Can you work these out from the model? Positions are in its coordinate system, mm. Face numbers are marked on the shaded views. A direction names the side the tool comes from. Give positions to 0.01 mm unless a question says otherwise; leave off trailing zeros. Loops run counter-clockwise (first coordinate to the right, second up) from the corner with the lowest first, then second, coordinate; pieces in that order, holes last. Notation, with made-up numbers: (9, -28) - (52, -28) arc R22 cw to (52, -1) - close; hole circle Ø4 at (72, 23.25). An arc over 180 degrees is marked (long way). Answer as a JSON object with one key per item and string values. Group by question number.
Item 1: Suppose I cut it at D-D on y = 0. Write out the boundary of the cut face in (x, z), and give its area (3 significant figures).
Item 2: Suppose I cut it at C-C on x = 15. Write out the boundary of the cut face in (y, z), and give its area (3 significant figures).
Item 3: Please list where these lines run through material, in increasing order: L1, parallel to X at y = 0, z = 2.35; L2, parallel to Y at x = 5, z = 2.25; L3, parallel to Z at x = 18, y = -3.25.
Item 4: Which directions (+Z, -Z, +X, -X, +Y, -Y) give clear straight access to the entire face, cutting with the end or side of a thin tool? Please do the marked faces 5 and 6.
Item 5: Suppose I cut it at A-A on y = 8.75. Write out the boundary of the cut face in (x, z), and give its area (3 significant figures).
Item 6: Thinking about a two-plate mould opening in X: for the marked faces 1, 2, 3 and 4, which applies, pulls with the +X half, pulls with the -X half, needs draft (parallel to the pull), parting line crosses it, or undercut?
Item 7: Will these pins go through, and if not, where does the flat tip stop? pin 1 (7 mm diameter, centred on x = -4.5, y = -5.5, fed in from +Z); pin 2 (2 mm diameter, centred on x = -19.5, y = -12, fed in from +Z).
Item 8: Suppose I cut it at B-B on z = 3.2. Write out the boundary of the cut face in (x, y).
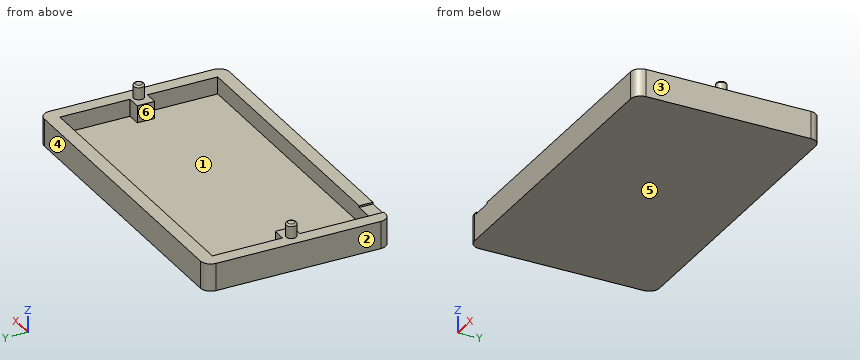
from build123d import *

# Parameters (mm, degrees)
SKETCH_W     = 46
SKETCH_H     = 27
PAD_DEPTH    = 2.5
SKETCH001_W  = 46
SKETCH001_H  = 27
PAD001_DEPTH = 1.5
SKETCH002_R  = 0.75
PAD002_DEPTH = 2
SKETCH003_W  = 3
SKETCH003_H  = 2
POCKET_DEPTH = 0.25
FILLET_R     = 0.25
FILLET001_R  = 1.5


with BuildPart() as part:
    # Sketch → Pad (new body)
    with BuildSketch(Plane.XY):
        Rectangle(SKETCH_W, SKETCH_H)
        Polygon((-21, 11.5), (21, 11.5), (21, 1.27), (19, 1.27), (19, -1.27), (21, -1.27), (21, -11.5), (-21, -11.5), (-21, -1.27), (-19, -1.27), (-19, 1.27), (-21, 1.27), align=None, mode=Mode.SUBTRACT)
    extrude(amount=PAD_DEPTH)

    # Sketch001 (on Face17 of Pad) → Pad001 (join)
    with BuildSketch(Plane(origin=(0, 0, 0), x_dir=(1, 0, 0), z_dir=(0, 0, -1))):
        Rectangle(SKETCH001_W, SKETCH001_H)
    extrude(amount=PAD001_DEPTH)

    # Sketch002 (on Face5 of Pad001) → Pad002 (join)
    with BuildSketch(Plane.XY.offset(2.5)):
        with Locations((-21, 0)):
            Circle(SKETCH002_R)
        with Locations((21, 0)):
            Circle(SKETCH002_R)
    extrude(amount=PAD002_DEPTH)

    # Sketch003 → Pocket (cut)
    with BuildSketch(Plane.XY.offset(2.5)):
        with Locations((-19.5, -12.5)):
            Rectangle(SKETCH003_W, SKETCH003_H)
    extrude(amount=-POCKET_DEPTH, mode=Mode.SUBTRACT)

    # Fillet
    fillet_edges = [part.edges().sort_by_distance(p)[0] for p in [
        (20.25, 0, 4.5),
        (-21.75, 0, 4.5),
    ]]
    fillet(fillet_edges, radius=FILLET_R)

    # Fillet001
    fillet001_edges = [part.edges().sort_by_distance(p)[0] for p in [
        (-23, -13.5, 1.25),
        (23, -13.5, 1.25),
        (-23, 13.5, 1.25),
        (23, 13.5, 1.25),
    ]]
    fillet(fillet001_edges, radius=FILLET001_R)


solid = part.part
Worked out:
{
 "1": {"outline": "(-23, -1.5) - (23, -1.5) - (23, 2.5) - (21.75, 2.5) - (21.75, 4.25) arc R0.25 ccw to (21.5, 4.5) - (20.5, 4.5) arc R0.25 ccw to (20.25, 4.25) - (20.25, 2.5) - (19, 2.5) - (19, 0) - (-19, 0) - (-19, 2.5) - (-20.25, 2.5) - (-20.25, 4.25) arc R0.25 ccw to (-20.5, 4.5) - (-21.5, 4.5) arc R0.25 ccw to (-21.75, 4.25) - (-21.75, 2.5) - (-23, 2.5) - close", "area": "94.9 mm2"},
 "2": {"outline": "(-13.5, -1.5) - (13.5, -1.5) - (13.5, 2.5) - (11.5, 2.5) - (11.5, 0) - (-11.5, 0) - (-11.5, 2.5) - (-13.5, 2.5) - close", "area": "50.5 mm2"},
 "3": {"L1": "x = -23 to -19, 19 to 23", "L2": "y = -13.5 to -11.5, 11.5 to 13.5", "L3": "z = -1.5 to 0"},
 "4": {"face 5": "-Z, +X, -X, +Y, -Y", "face 6": "+Z"},
 "5": {"outline": "(-23, -1.5) - (23, -1.5) - (23, 2.5) - (21, 2.5) - (21, 0) - (-21, 0) - (-21, 2.5) - (-23, 2.5) - close", "area": "79.0 mm2"},
 "6": {"face 1": "undercut", "face 2": "pulls with the -X half", "face 3": "pulls with the +X half", "face 4": "needs draft"},
 "7": {"pin 1": "stops at z = 0", "pin 2": "stops at z = 2.25"},
 "8": {"outline": "circle Ø1.5 at (-21, 0); circle Ø1.5 at (21, 0)"}
}
